Can you work these out from the model? Positions are in its coordinate system, mm. Coordinates: 2 decimals unless noted, no trailing zeros. Loops run counter-clockwise (first coordinate to the right, second up) from the corner with the lowest first, then second, coordinate; pieces in that order, holes last. Notation, with made-up numbers: (66, 66) -> (88, 66) arc R24 cw to (88, 82) -> close; hole circle Ø11 at (-26, 39). An arc over 180 degrees is marked (long way). Use one line per item in the form item = value. Start each with the question number.
(1) I'm going to push flat-ended pins straight in: pin 1 (7 mm diameter, centred on x = -32.5, z = -14, fed in from +Y); pin 2 (4 mm diameter, centred on x = -5.5, z = -0.5, fed in from -Y). Where does each tip first touch, or does it pass through?
(2) Imagine slicing it at A-A (z = 14). List the corners of the cut face in (x, y) for me.
(3) Imagine slicing it at B-B (x = -32.5). List the corners of the cut face in (y, z) for me.
(4) I need wall thicknesses on line 1 (X direction, y = 1.4, z = -14); line 2 (Z direction, x = -32.5, y = 1.25); line 3 (Y direction, x = -32.5, z = -18.5). Which ranges of each line are inside material? Lowest first, please. Write a range as [from, to].
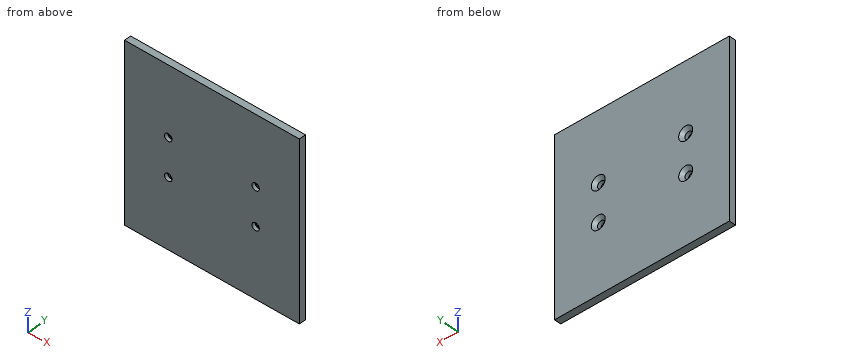
```python
from build123d import *

# Parameters (mm, degrees)
SCHIZZO1_W                            = 130
SCHIZZO1_H                            = 130
ESTRUSIONE_ESTRUSIONE1_DEPTH          = 5
FORO_SVASATO_PER_VITE_M5_1_AT_2_COUNT = 2
FORO_SVASATO_PER_VITE_M5_1_AT_2_PITCH = 65
FORO_SVASATO_PER_VITE_M5_1_AT_3_COUNT = 2
FORO_SVASATO_PER_VITE_M5_1_AT_3_PITCH = 70.774289117
FORO_SVASATO_PER_VITE_M5_1_AT_4_COUNT = 2
FORO_SVASATO_PER_VITE_M5_1_AT_4_PITCH = 28


with BuildPart() as part:
    # Schizzo1 → Estrusione-Estrusione1 (new body)
    with BuildSketch(Plane(origin=(0, 0, 0), x_dir=(1, 0, 0), z_dir=(0, 1, 0))):
        Rectangle(SCHIZZO1_W, SCHIZZO1_H)
    extrude(amount=ESTRUSIONE_ESTRUSIONE1_DEPTH)

    # Schizzo4 → Foro svasato per Vite M5-1 (revolve, cut)
    with BuildSketch(Plane(origin=(-32.5, 5, -14), x_dir=(0, 0, 1), z_dir=(1, 0, 0))):
        Polygon((0, 0), (0, 5), (2.75, 5), (2.75, 2.45), (5.2, 0), align=None)
    foro_svasato_per_vite_m5_1 = revolve(axis=Axis((-32.5, 11.35, -14), (0, -1, 0)), mode=Mode.SUBTRACT)

    # Foro svasato per Vite M5-1 at 2: Foro svasato per Vite M5-1 ×2
    with Locations(*[(i * FORO_SVASATO_PER_VITE_M5_1_AT_2_PITCH, 0, 0) for i in range(1, FORO_SVASATO_PER_VITE_M5_1_AT_2_COUNT)]):
        add(foro_svasato_per_vite_m5_1, mode=Mode.SUBTRACT)

    # Foro svasato per Vite M5-1 at 3: Foro svasato per Vite M5-1 ×2
    with Locations(*[Vector(0.9184126158110061, 0, 0.39562389604166415) * (i * FORO_SVASATO_PER_VITE_M5_1_AT_3_PITCH) for i in range(1, FORO_SVASATO_PER_VITE_M5_1_AT_3_COUNT)]):
        add(foro_svasato_per_vite_m5_1, mode=Mode.SUBTRACT)

    # Foro svasato per Vite M5-1 at 4: Foro svasato per Vite M5-1 ×2
    with Locations(*[(0, 0, i * FORO_SVASATO_PER_VITE_M5_1_AT_4_PITCH) for i in range(1, FORO_SVASATO_PER_VITE_M5_1_AT_4_COUNT)]):
        add(foro_svasato_per_vite_m5_1, mode=Mode.SUBTRACT)


solid = part.part
```
Worked out:
q1.pin_1 = 3.3
q1.pin_2 = 0
q2.outline = (-65, 0) -> (-35.25, 0) -> (-35.25, 2.55) -> (-37.7, 5) -> (-65, 5) -> close; (-29.75, 0) -> (29.75, 0) -> (29.75, 2.55) -> (27.3, 5) -> (-27.3, 5) -> (-29.75, 2.55) -> close; (35.25, 0) -> (65, 0) -> (65, 5) -> (37.7, 5) -> (35.25, 2.55) -> close
q3.outline = (0, -65) -> (5, -65) -> (5, -19.2) -> (2.55, -16.75) -> (0, -16.75) -> close; (0, -11.25) -> (2.55, -11.25) -> (5, -8.8) -> (5, 8.8) -> (2.55, 11.25) -> (0, 11.25) -> close; (0, 16.75) -> (2.55, 16.75) -> (5, 19.2) -> (5, 65) -> (0, 65) -> close
q4.line_1 = [-65, -35.25], [-29.75, 29.75], [35.25, 65]
q4.line_2 = [-65, -16.75], [-11.25, 11.25], [16.75, 65]
q4.line_3 = [0, 4.3]
